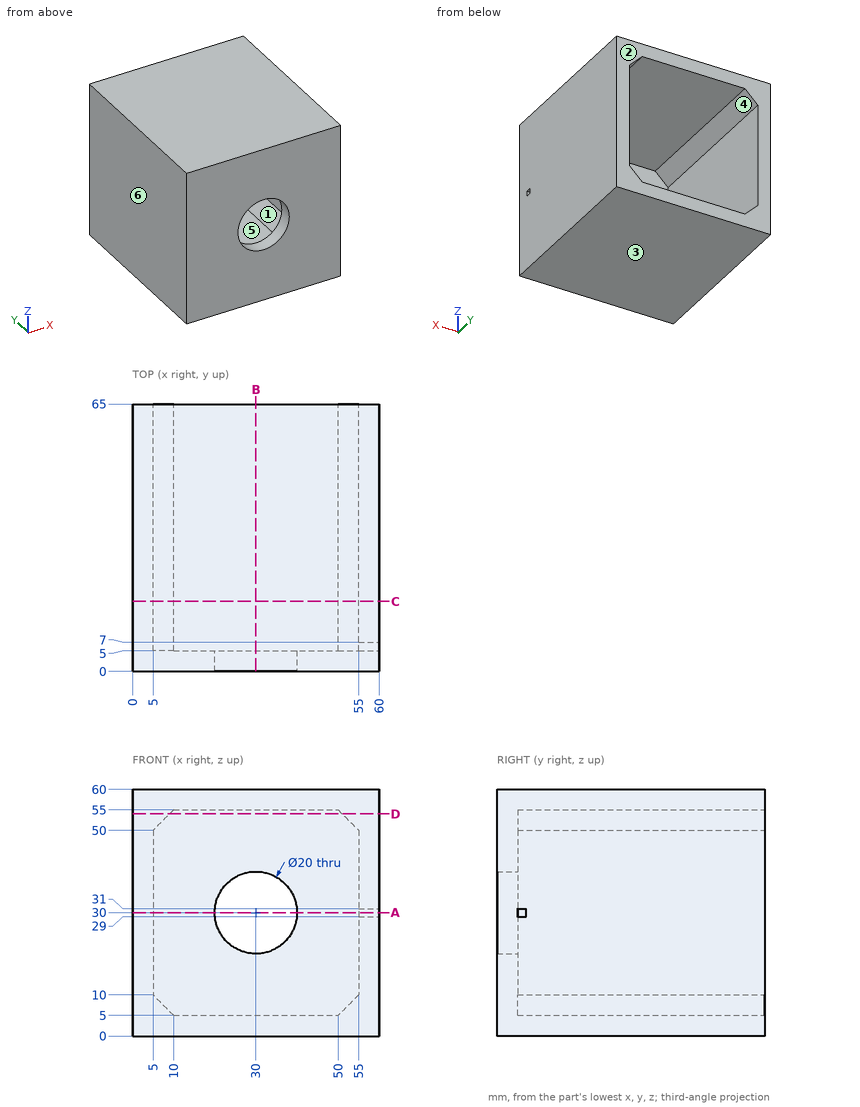
Geometry check sheet. Reference: drawing and pictorial views, mm from the part's lowest x, y, z. A direction names the side the tool comes from. Round coordinates to 2 decimals unless told otherwise and drop trailing zeros. Loops run counter-clockwise (first coordinate to the right, second up) from the corner with the lowest first, then second, coordinate; pieces in that order, holes last. Notation, with made-up numbers: (-29.75, 85) - (22.25, 85) arc R28 ccw to (22.25, 110) - close; hole circle Ø7 at (42, 8). An arc over 180 degrees is marked (long way). Answer in a Markdown table with one row per item. Add a question column.
Q1. Tool access check on the marked faces 1 and 2. Record the directions out of +Z, -Z, +X, -X, +Y, -Y that give a thin tool (end or side, any length) a straight path to the whole face; none if there is none.
Q2. Gauge pin test, flat ends, axial feed: pin 1 (5 mm diameter, centred on x = 21, z = 37.5, fed in from +Y); pin 2 (12 mm diameter, centred on x = 30, z = 30, fed in from -Y). Record the tip position at first contact, or that the pin passes through.
Q3. Release check for a two-part mould opening along Z. For the marked faces 3, 4, 5 and 6 record: pulls with the +Z half, pulls with the -Z half, needs draft (parallel to the pull), parting line crosses it, or undercut.
Q4. Material ranges on line 1 (X direction, y = 2.2, z = 30); line 2 (Z direction, x = 24, y = 28.5), recorded low to high.
Q5. Section check A-A on z = 30. Enter the section's corners in (x, y), plus the area to 3 significant figures.
Q6. Section check B-B on x = 30. Enter the section's corners in (y, z), plus the area to 3 significant figures.
Q7. Section check D-D on z = 54. Enter the section's corners in (x, y), plus the area to 3 significant figures.
Q8. Section check C-C on y = 17. Enter the section's corners in (x, z), plus the area to 3 significant figures.
Found:
| question | item | result |
|---|---|---|
| 1 | face 1 | +Y |
| 1 | face 2 | +Z, -Z, +X, -X, +Y |
| 2 | pin 1 | stops at y = 5 |
| 2 | pin 2 | passes through |
| 3 | face 3 | pulls with the -Z half |
| 3 | face 4 | undercut |
| 3 | face 5 | undercut |
| 3 | face 6 | needs draft |
| 4 | line 1 | x = 0 to 20, 40 to 60 |
| 4 | line 2 | z = 0 to 5, 55 to 60 |
| 5 | outline | (0, 0) - (20, 0) - (20, 5) - (5, 5) - (5, 65) - (0, 65) - close; (40, 0) - (60, 0) - (60, 5) - (40, 5) - close; (55, 7) - (60, 7) - (60, 65) - (55, 65) - close |
| 5 | area | 790 mm² |
| 6 | outline | (0, 0) - (65, 0) - (65, 5) - (5, 5) - (5, 20) - (0, 20) - close; (0, 40) - (5, 40) - (5, 55) - (65, 55) - (65, 60) - (0, 60) - close |
| 6 | area | 800 mm² |
| 7 | outline | (0, 0) - (60, 0) - (60, 65) - (51, 65) - (51, 5) - (9, 5) - (9, 65) - (0, 65) - close |
| 7 | area | 1,380 mm² |
| 8 | outline | (0, 0) - (60, 0) - (60, 60) - (0, 60) - close; hole (5, 10) - (10, 5) - (50, 5) - (55, 10) - (55, 50) - (50, 55) - (10, 55) - (5, 50) - close |
| 8 | area | 1,150 mm² |
